```python
from build123d import *

# Parameters (mm, degrees)
SKETCH2_R           = 21.5
SKETCH2_R_2         = 1.5
SKETCH2_R_3         = 1.499999999
BOSS_EXTRUDE1_DEPTH = 4
SKETCH4_R           = 2.75
CUT_EXTRUDE1_DEPTH  = 2.5
SKETCH6_R           = 6.5
BOSS_EXTRUDE2_DEPTH = 15
SKETCH8_R           = 3
CUT_EXTRUDE2_DEPTH  = 61
SKETCH9_R           = 1.5
CUT_EXTRUDE3_DEPTH  = 8
SKETCH11_R          = 1.5
CUT_EXTRUDE5_DEPTH  = 29.064832946


with BuildPart() as part:
    # Sketch2 → Boss-Extrude1 (new body)
    with BuildSketch(Plane.XY):
        with Locations((4.706896552, 17.280444568)):
            Circle(SKETCH2_R)
        with Locations((-8.895989131, 29.060889133)):
            Circle(SKETCH2_R_2, mode=Mode.SUBTRACT)
        with Locations((18.309782235, 29.060889133)):
            Circle(SKETCH2_R_3, mode=Mode.SUBTRACT)
        with Locations((1.706896552, 5.5)):
            Circle(SKETCH2_R_2, mode=Mode.SUBTRACT)
        with Locations((7.706896552, 5.5)):
            Circle(SKETCH2_R_2, mode=Mode.SUBTRACT)
    extrude(amount=BOSS_EXTRUDE1_DEPTH)

    # Sketch4 → Cut-Extrude1 (cut)
    with BuildSketch(Plane.XY.offset(4)):
        with Locations((-8.895989131, 29.060889133)):
            Circle(SKETCH4_R)
        with Locations((18.309782235, 29.060889133)):
            Circle(SKETCH4_R)
        with Locations((7.706896552, 5.5)):
            Circle(SKETCH4_R)
        with Locations((1.706896552, 5.5)):
            Circle(SKETCH4_R)
    extrude(amount=-CUT_EXTRUDE1_DEPTH, mode=Mode.SUBTRACT)

    # Sketch6 → Boss-Extrude2 (add)
    with BuildSketch(Plane.XY.offset(4)):
        with Locations((4.706896552, 17.280444568)):
            Circle(SKETCH6_R)
    extrude(amount=BOSS_EXTRUDE2_DEPTH)

    # Sketch8 → Cut-Extrude2 (cut)
    with BuildSketch(Plane.XY.offset(19)):
        with Locations((4.706896552, 17.280444568)):
            Circle(SKETCH8_R)
    extrude(amount=-CUT_EXTRUDE2_DEPTH, mode=Mode.SUBTRACT)

    # Sketch9 → Cut-Extrude3 (cut)
    with BuildSketch(Plane.XY.offset(19)):
        with Locations((4.706896552, 22.030444568)):
            Circle(SKETCH9_R)
        with Locations((9.456896552, 17.280444568)):
            Circle(SKETCH9_R)
        with Locations((4.706896552, 12.530444568)):
            Circle(SKETCH9_R)
        with Locations((-0.043103448, 17.280444568)):
            Circle(SKETCH9_R)
    extrude(amount=-CUT_EXTRUDE3_DEPTH, mode=Mode.SUBTRACT)

    # Sketch11 → Cut-Extrude5 (cut)
    with BuildSketch(Plane(origin=(0, 0, 0), x_dir=(1, 0, 0), z_dir=(0, 1, 0))):
        with Locations(Location((4.706896552, -16, 0), (0, 0, 90))):
            Circle(SKETCH11_R)
        with Locations(Location((4.706896552, -11, 0), (0, 0, 90))):
            Circle(SKETCH11_R)
    extrude(amount=CUT_EXTRUDE5_DEPTH, mode=Mode.SUBTRACT)


solid = part.part
```
Model file for the job. Use its own axes, mm. A direction names the side the tool comes from. Coordinates: 2 decimals unless noted, no trailing zeros. Order: outer loops, then holes, each group sorted by start corner. A loop starts at its lowest first (then second) coordinate and runs counter-clockwise, first axis right, second up. Notation, with made-up numbers: (68, 50) -> (124, 50) arc R21 cw to (124, 61) -> close; hole circle Ø5 at (3.5, -38). An arc over 180 degrees is marked (long way). Answer as a JSON object with one key per item and string values. Group by question number.
1) Which spindle directions (+Z, -Z, +X, -X, +Y, -Y) get a long thin tool onto all of the face, cutting with end or side? Do faces 1 (the face through (1.111, 2.815, 2.768)), 2 (the face through (6.517, 4.587, 0.74)). Say none if no direction does.
2) Cut at A-A, the plane y = 5.5. Write the cut outline in (x, z).
3) Cut at C-C, the plane y = 0. Write the cut outline in (x, z), then the cut area to 3 significant figures.
4) Cut at B-B, the plane z = 8.5. Write the cut outline in (x, y).
5) Flat gauge pins, fed straight in: pin 1 (7 mm diameter, centred on x = 18.31, y = 29.06, fed in from +Z); pin 2 (1 mm diameter, centred on x = 10, y = 7.5, fed in from -Z); pin 3 (8 mm diameter, centred on y = 32.5, z = 4, fed in from -X); pin 4 (1.5 mm diameter, centred on y = 29, z = 3, fed in from -X). Where does each tip first touch, or does it go through?
6) Cut at D-D, the plane x = -14. Write the cut outline in (y, z).
7) Pull direction Z, two halves, no side cores. Call faces 3 (the face through (3.093, 4.925, 0.74)), 4 (the face through (3.22, 23.29, 16.2)), 5 (the face through (-7.7, 27.9, 1.5)): +Z half, -Z half, draft (parallel to the pull), parting line (faces both ways), or undercut.
8) Drill centre lines: L1, parallel to X at y = 6, z = 3.5; L2, parallel to X at y = 5.5, z = 1.1; L3, parallel to Z at x = -4.5, y = 5.5. Where is each one in solid material? Low to high.
Check values:
{
 "1": {"face 1": "+Z", "face 2": "+Z, -Z"},
 "2": {"outline": "(-13.28, 0) -> (0.21, 0) -> (0.21, 1.5) -> (-1.04, 1.5) -> (-1.04, 4) -> (-13.28, 4) -> close; (3.21, 0) -> (6.21, 0) -> (6.21, 1.5) -> (4.96, 1.5) -> (4.96, 4) -> (4.46, 4) -> (4.46, 1.5) -> (3.21, 1.5) -> close; (9.21, 0) -> (22.69, 0) -> (22.69, 4) -> (10.46, 4) -> (10.46, 1.5) -> (9.21, 1.5) -> close"},
 "3": {"outline": "(-8.09, 0) -> (17.5, 0) -> (17.5, 4) -> (-8.09, 4) -> close", "area": "102 mm²"},
 "4": {"outline": "circle Ø13 at (4.71, 17.28); hole circle Ø6 at (4.71, 17.28)"},
 "5": {"pin 1": "stops at z = 4", "pin 2": "stops at z = 0", "pin 3": "stops at x = -13.63", "pin 4": "stops at x = -13.78"},
 "6": {"outline": "(6.68, 0) -> (27.88, 0) -> (27.88, 4) -> (6.68, 4) -> close"},
 "7": {"face 3": "draft", "face 4": "undercut", "face 5": "+Z half"},
 "8": {"L1": "x = -13.6 to -1, 4.41 to 5, 10.41 to 23.01", "L2": "x = -13.28 to 0.21, 3.21 to 6.21, 9.21 to 22.69", "L3": "z = 0 to 4"}
}
